```python
from build123d import *

# Parameters (mm, degrees)
F1_DEPTH = 25
F2_R     = 10
F3_DEPTH = 15


with BuildPart() as f1:
    # F0 (on Top) → F1 (new body)
    with BuildSketch(Plane.XY):
        Polygon((0, 32.679492), (0, 0), (60, 0), (60, 50), (30, 50), align=None)
    extrude(amount=F1_DEPTH)

    # F2 (on face) → F3 (cut)
    with BuildSketch(Plane.XY.offset(25)):
        with Locations((30, 20)):
            Circle(F2_R)
    extrude(amount=-F3_DEPTH, mode=Mode.SUBTRACT)


solid = f1.part
```
Model file for the job. Use its own axes, mm. Coordinates: 2 decimals unless noted, no trailing zeros. Loops run counter-clockwise (first coordinate to the right, second up) from the corner with the lowest first, then second, coordinate; pieces in that order, holes last. Notation, with made-up numbers: M 23.25,-22 L 50.25,-22 A35 cw 50.25,10 Z; hole C 2,62 d1. An arc over 180 degrees is marked long. Use CSV: the item, a comma, the result in double quotes. Start each with the question number.
1. Band-saw the part on D-D, the plane x = 39. List the corners of the cut face in (y, z), then the cut area to 3 significant figures.
2. Probe probe 1 along Y at (x, z) = (30, 16); probe 2 along Z at (x, y) = (21.5, 15.5); probe 3 along Y at (x, z) = (15, 22.5). List the from-to ranges inside material, lowest first. Write a range as [from, to].
3. Band-saw the part on B-B, the plane y = 20. List the corners of the cut face in (x, z).
4. Band-saw the part on A-A, the plane z = 22. List the corners of the cut face in (x, y).
5. Band-saw the part on C-C, the plane z = 7. List the corners of the cut face in (x, y), then the cut area to 3 significant figures.
6. Flat gauge pins, fed straight in: pin 1 (8 mm diameter, centred on x = 29, y = 25.5, fed in from -Z); pin 2 (16 mm diameter, centred on x = 30, y = 20, fed in from +Z); pin 3 (6 mm diameter, centred on x = 24.5, z = 13, fed in from +Y); pin 4 (12 mm diameter, centred on x = 17, z = 18.5, fed in from +Y). Where does each tip first touch, or does it go through?
7. Two-plate mould, pull along X, no slides. Class faces 1 (the flat face through (30, 20, 10)), 2 (the flat face through (30, 25, 0)), 3 (the cylindrical face through (39.54, 23, 17.6)), 4 (the flat face through (60, 25, 12)): pulls with the +X half, pulls with the -X half, needs draft (parallel to the pull), parting line crosses it, or undercut.
Entries:
1,outline,"M 0,0 L 50,0 L 50,25 L 24.36,25 L 24.36,10 L 15.64,10 L 15.64,25 L 0,25 Z"
1,area,"1,120 mm2"
2,probe 1,"y = [0, 10], [30, 50]"
2,probe 2,"z = [0, 10]"
2,probe 3,"y = [0, 41.34]"
3,outline,"M 0,0 L 60,0 L 60,25 L 40,25 L 40,10 L 20,10 L 20,25 L 0,25 Z"
4,outline,"M 0,0 L 60,0 L 60,50 L 30,50 L 0,32.68 Z; hole C 30,20 d20"
5,outline,"M 0,0 L 60,0 L 60,50 L 30,50 L 0,32.68 Z"
5,area,"2,740 mm2"
6,pin 1,"stops at z = 0"
6,pin 2,"stops at z = 10"
6,pin 3,"stops at y = 48.56"
6,pin 4,"stops at y = 45.96"
7,face 1,"undercut"
7,face 2,"needs draft"
7,face 3,"undercut"
7,face 4,"pulls with the +X half"
